from build123d import *

# Parameters (mm, degrees)
CUT_EXTRUDE1_DEPTH   = 5
CUT_EXTRUDE3_DEPTH   = 45
SKETCH8_R            = 40
CUT_EXTRUDE4_DEPTH   = 32
SKETCH9_R            = 32
SKETCH9_R_2          = 24.5
CUT_EXTRUDE5_DEPTH   = 14
SKETCH10_R           = 26
CUT_EXTRUDE6_DEPTH   = 14
FILLET1_R            = 7
FILLET2_R            = 7
CUT_REVOLVE1_START   = 22
CUT_REVOLVE1_DEPTH   = 30.5
CUT_EXTRUDE12_DEPTH  = 5
SKETCH18_W           = 13
SKETCH18_H           = 8
CUT_EXTRUDE13_DEPTH  = 5
INTERSECT1_OUTLINE_R = 42
INTERSECT1_DEPTH     = 55
SKETCH20_W           = 10
SKETCH20_H           = 5
BOSS_EXTRUDE1_DEPTH  = 13
BOSS_EXTRUDE3_DEPTH  = 7
SKETCH19_R           = 1.5
CUT_EXTRUDE14_DEPTH  = 20
SKETCH23_W           = 20
SKETCH23_H           = 7
CUT_EXTRUDE15_DEPTH  = 7
SKETCH24_W           = 44
SKETCH24_H           = 3.5
CUT_EXTRUDE16_DEPTH  = 5
SKETCH25_R           = 2.75
CUT_EXTRUDE17_DEPTH  = 5
FILLET4_R            = 3
FILLET6_R            = 4


with BuildPart() as part:
    # Sketch1 → Revolve1 (revolve)
    with BuildSketch(Plane.XY, mode=Mode.PRIVATE) as revolve1_sk:
        with BuildLine():
            Line((22.5, 0), (32, 0))
            ThreePointArc((32, 0), (33.414213562, 0.585786438), (34, 2))
            Line((34, 2), (34, 18))
            Line((34, 18), (40, 18))
            ThreePointArc((40, 18), (41.414213562, 18.585786438), (42, 20))
            Line((42, 20), (42, 55))
            ThreePointArc((42, 55), (40.535533906, 58.535533906), (37, 60))
            Line((37, 60), (0, 60))
            Line((0, 60), (0, 18))
            Line((0, 18), (22.5, 18))
            Line((22.5, 18), (22.5, 0))
        make_face()
    revolve(revolve1_sk.sketch.rotate(Axis((0, 2, 0), (0, 1, 0)), 90), axis=Axis((0, 2, 0), (0, 1, 0)))

    # Sketch5 → Cut-Extrude1 (cut)
    with BuildSketch(Plane(origin=(0, 60, 0), x_dir=(1, 0, 0), z_dir=(0, 1, 0))):
        with BuildLine():
            Line((-42, 0), (-40, 0))
            Line((-40, 0), (40, 0))
            Line((40, 0), (42, 0))
            ThreePointArc((42, 0), (0, 42), (-42, 0))
        make_face()
    extrude(amount=-CUT_EXTRUDE1_DEPTH, mode=Mode.SUBTRACT)

    # Sketch7 → Cut-Extrude3 (cut)
    with BuildSketch(Plane.XZ.offset(-18)):
        with BuildLine():
            Line((-21, 0), (21, 0))
            ThreePointArc((21, 0), (0, -21), (-21, 0))
        make_face()
    extrude(amount=-CUT_EXTRUDE3_DEPTH, mode=Mode.SUBTRACT)

    # Sketch8 → Cut-Extrude4 (cut)
    with BuildSketch(Plane(origin=(0, 52.5, 0), x_dir=(1, 0, 0), z_dir=(0, 1, 0))):
        with Locations(Location((0, 0, 0), (0, 0, 270))):
            Circle(SKETCH8_R)
        with BuildLine():
            Line((22.912878475, -2), (-22.912878475, -2))
            ThreePointArc((-22.912878475, -2), (0, 23), (22.912878475, -2))
        make_face(mode=Mode.SUBTRACT)
    extrude(amount=-CUT_EXTRUDE4_DEPTH, mode=Mode.SUBTRACT)

    # Sketch9 → Cut-Extrude5 (cut)
    with BuildSketch(Plane(origin=(0, 2, 0), x_dir=(-1, 0, 0), z_dir=(0, -1, 0))):
        with Locations(Location((0, 0, 0), (0, 0, 90))):
            Circle(SKETCH9_R)
        with Locations(Location((0, 0, 0), (0, 0, 90))):
            Circle(SKETCH9_R_2, mode=Mode.SUBTRACT)
    extrude(amount=-CUT_EXTRUDE5_DEPTH, mode=Mode.SUBTRACT)

    # Sketch10 → Cut-Extrude6 (cut)
    with BuildSketch(Plane(origin=(0, 2, 0), x_dir=(-1, 0, 0), z_dir=(0, -1, 0))):
        Circle(SKETCH10_R)
    extrude(amount=-CUT_EXTRUDE6_DEPTH, mode=Mode.SUBTRACT)

    # Fillet1
    fillet1_edges = [part.edges().sort_by_distance(p)[0] for p in [
        (21, 36.5, 0),
        (-21, 36.5, 0),
    ]]
    fillet(fillet1_edges, radius=FILLET1_R)

    # Fillet2
    fillet2_edges = [part.edges().sort_by_distance(p)[0] for p in [
        (-22.912878475, 36.5, 2),
        (22.912878475, 36.5, 2),
    ]]
    fillet(fillet2_edges, radius=FILLET2_R)

    # Cut-Revolve1: read off the stored shape, not the designer's step
    # Cut-Revolve1 outline → Cut-Revolve1 (cut)
    with BuildSketch(Plane(origin=(0, 0, 0), x_dir=(1, 0, 0), z_dir=(0, 1, 0)).offset(CUT_REVOLVE1_START)):
        with BuildLine():
            Line((-34.641016151, -20), (-36.373066959, -21))
            ThreePointArc((-36.373066959, -21), (0, -42), (36.373066959, -21))
            Line((36.373066959, -21), (34.641016151, -20))
            ThreePointArc((34.641016151, -20), (0, -40), (-34.641016151, -20))
        make_face()
    extrude(amount=CUT_REVOLVE1_DEPTH, mode=Mode.SUBTRACT)

    # Sketch15 → Cut-Extrude12 (cut)
    with BuildSketch(Plane(origin=(0, 20.5, 0), x_dir=(1, 0, 0), z_dir=(0, 1, 0))):
        with BuildLine():
            Line((-28.124355653, -3.514579578), (-26.124355653, -3.514579578))
            ThreePointArc((-26.124355653, -3.514579578), (-24.710142091, -2.928793141), (-24.124355653, -1.514579578))
            Line((-24.124355653, -1.514579578), (-24.124355653, 8.485420422))
            ThreePointArc((-24.124355653, 8.485420422), (-24.710142091, 9.899633984), (-26.124355653, 10.485420422))
            Line((-26.124355653, 10.485420422), (-28.124355653, 10.485420422))
            ThreePointArc((-28.124355653, 10.485420422), (-29.538569215, 9.899633984), (-30.124355653, 8.485420422))
            Line((-30.124355653, 8.485420422), (-30.124355653, -1.514579578))
            ThreePointArc((-30.124355653, -1.514579578), (-29.538569215, -2.928793141), (-28.124355653, -3.514579578))
        make_face()
    extrude(amount=-CUT_EXTRUDE12_DEPTH, mode=Mode.SUBTRACT)

    # Sketch18 → Cut-Extrude13 (cut)
    with BuildSketch(Plane(origin=(0, 55, 0), x_dir=(1, 0, 0), z_dir=(0, 1, 0))):
        with Locations((0.796512215, 32.951769165)):
            Rectangle(SKETCH18_W, SKETCH18_H)
    extrude(amount=-CUT_EXTRUDE13_DEPTH, mode=Mode.SUBTRACT)

    # Intersect1: read off the stored shape, not the designer's step
    # Intersect1 outline → Intersect1 (cut)
    with BuildSketch(Plane(origin=(0, 0, 0), x_dir=(1, 0, 0), z_dir=(0, 1, 0))):
        Circle(INTERSECT1_OUTLINE_R)
        with BuildLine():
            Line((12.124355653, 0), (-12.124355653, 0))
            ThreePointArc((-12.124355653, 0), (-18.186533479, 3.5), (-18.186533479, 10.5))
            ThreePointArc((-18.186533479, 10.5), (0, 21), (18.186533479, 10.5))
            ThreePointArc((18.186533479, 10.5), (18.186533479, 3.5), (12.124355653, 0))
        make_face(mode=Mode.SUBTRACT)
    extrude(amount=INTERSECT1_DEPTH, mode=Mode.SUBTRACT)

    # Sketch20 → Boss-Extrude1 (add)
    with BuildSketch(Plane.XZ.offset(-55)):
        with Locations((0, 30)):
            Rectangle(SKETCH20_W, SKETCH20_H)
    extrude(amount=BOSS_EXTRUDE1_DEPTH)

    # Sketch22 → Boss-Extrude3 (add)
    with BuildSketch(Plane(origin=(0, 0, 0), x_dir=(-1, 0, 0), z_dir=(0, 0, -1))):
        with BuildLine():
            Line((-42, 55), (42, 55))
            ThreePointArc((42, 55), (40.535533906, 58.535533906), (37, 60))
            Line((37, 60), (-37, 60))
            ThreePointArc((-37, 60), (-40.535533906, 58.535533906), (-42, 55))
        make_face()
    extrude(amount=BOSS_EXTRUDE3_DEPTH)

    # Sketch19 → Cut-Extrude14 (cut)
    with BuildSketch(Plane(origin=(0, 0, -7), x_dir=(-1, 0, 0), z_dir=(0, 0, -1))):
        with Locations((0, 57.5)):
            Circle(SKETCH19_R)
        with Locations((-29.45, 57.5)):
            Circle(SKETCH19_R)
        with Locations((29.45, 57.5)):
            Circle(SKETCH19_R)
    extrude(amount=-CUT_EXTRUDE14_DEPTH, mode=Mode.SUBTRACT)

    # Sketch23 → Cut-Extrude15 (cut)
    with BuildSketch(Plane(origin=(0, 60, 0), x_dir=(1, 0, 0), z_dir=(0, 1, 0))):
        with Locations((-32, 3.5)):
            Rectangle(SKETCH23_W, SKETCH23_H)
        with Locations((32, 3.5)):
            Rectangle(SKETCH23_W, SKETCH23_H)
    extrude(amount=-CUT_EXTRUDE15_DEPTH, mode=Mode.SUBTRACT)

    # Sketch24 → Cut-Extrude16 (cut)
    with BuildSketch(Plane(origin=(0, 60, 0), x_dir=(1, 0, 0), z_dir=(0, 1, 0))):
        with Locations((0, 5.25)):
            Rectangle(SKETCH24_W, SKETCH24_H)
    extrude(amount=-CUT_EXTRUDE16_DEPTH, mode=Mode.SUBTRACT)

    # Sketch25 → Cut-Extrude17 (cut)
    with BuildSketch(Plane(origin=(0, 0, 27.5), x_dir=(-1, 0, 0), z_dir=(0, 0, -1))):
        with Locations((0, 46.8)):
            Circle(SKETCH25_R)
    extrude(amount=-CUT_EXTRUDE17_DEPTH, mode=Mode.SUBTRACT)

    # Fillet4
    # the kernel refuses this fillet: 3 mm, written as the material it takes off along each edge
    with BuildSketch(Plane(origin=(12.5, 42, 27.5), x_dir=(0, 1, 0), z_dir=(-1, 0, 0))) as fillet4_piece_1:
        with BuildLine():
            CenterArc((FILLET4_R, -FILLET4_R), FILLET4_R, 90, 90)
            Line((0, -FILLET4_R), (0, 0))
            Line((0, 0), (FILLET4_R, 0))
        make_face()
    extrude(amount=25, mode=Mode.SUBTRACT)

    # Fillet6
    # the kernel refuses this fillet: 4 mm, written as the material it takes off along each edge
    with BuildSketch(Plane(origin=(-13.660254038, 42, 32.5), x_dir=(0, 1, 0), z_dir=(1, 0, 0))) as fillet6_piece_1:
        with BuildLine():
            CenterArc((3.464101615, -4), FILLET6_R, 90, 60)
            Line((0, -2), (0, 0))
            Line((0, 0), (3.464101615, 0))
        make_face()
    extrude(amount=27.320508076, mode=Mode.SUBTRACT)


solid = part.part
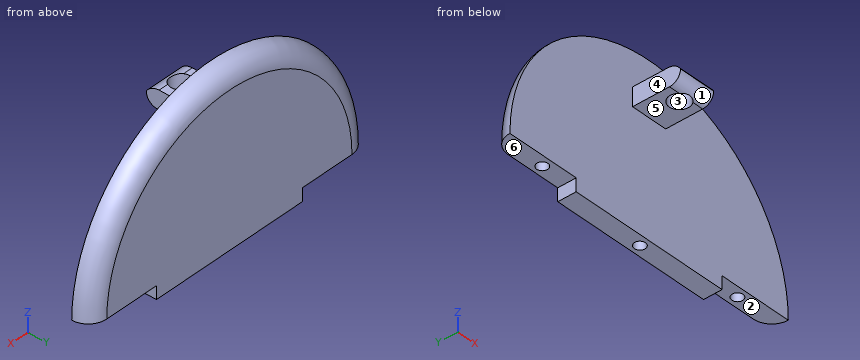
The model under review builds one solid part; all positions refer to its coordinate system, in mm. Face numbers are marked on the shaded views. A direction names the side the tool comes from. Round coordinates to 2 decimals unless told otherwise and drop trailing zeros. Loops run counter-clockwise (first coordinate to the right, second up) from the corner with the lowest first, then second, coordinate; pieces in that order, holes last. Notation, with made-up numbers: (83, -9.75) -> (133, -9.75) arc R16 cw to (133, -5.75) -> close; hole circle Ø5 at (-26.5, -9). An arc over 180 degrees is marked (long way). Answer as CSV lines item,"result".
1) Add section C-C on z = 9.5. State how many separate pieces and enclosed holes the cut face has, plus the area to 3 significant figures.
Geometry results:
separate pieces,"1"
enclosed holes,"3"
area,"377 mm²"
2) To check wall thickness, follow line 1 along Y through (x, z) = (0, 9); line 2 along Y through (x, z) = (-23, 12); line 3 along Y through (x, z) = (0, 29). State the ranges of each line that lie inside material, in increasing order. Write a range as from..to.
Geometry results:
line 1,"y = 55..56, 59..60"
line 2,"y = 55..60"
line 3,"y = 42.4..44.05, 49.55..60"
3) Add section A-A on y = 46.8. Write out the cut boundary in (x, z), plus the area to 3 significant figures.
Geometry results:
outline,"(-5, 27.5) -> (-2.75, 27.5) -> (-2.75, 32.5) -> (-5, 32.5) -> close; (2.75, 27.5) -> (5, 27.5) -> (5, 32.5) -> (2.75, 32.5) -> close"
area,"22.5 mm²"
4) Add section B-B on y = 52.75. Write out the cut boundary in (x, z), plus the area to 3 significant figures.
Geometry results:
outline,"(-5, 27.5) -> (5, 27.5) -> (5, 32.5) -> (-5, 32.5) -> close"
area,"50.0 mm²"
5) Tool access review of the marked faces 4, 5 and 6: name each direction out of +Z, -Z, +X, -X, +Y, -Y from which nothing blocks a thin tool from reaching the whole face with its end or side.
Geometry results:
face 4,"+Z, -Z, -X, -Y"
face 5,"-Z, +X, -X, -Y"
face 6,"-Z, -X, +Y, -Y"
6) For P1, Ø7, axis at x = 0, y = 46.8, coming from the +Z side; P2, Ø2.5, axis at y = 50, z = 30.5, coming from the -X side; P3, Ø2.5, axis at x = -30.5, y = 56.5, coming from the -Z side; P4, Ø5, axis at y = 50.5, z = 2.5, coming from the -X side, all flat-tipped, find the tip position at first contact; note any pin that passes through.
Geometry results:
P1,"stops at z = 32.5"
P2,"stops at x = -5"
P3,"stops at z = 0"
P4,"passes through"
7) Draft analysis for pull direction Y (two halves, no side actions). For the marked faces 1, 2 and 3, state which applies: pulls with the +Y half, pulls with the -Y half, needs draft (parallel to the pull), parting line crosses it, or undercut.
Geometry results:
face 1,"pulls with the -Y half"
face 2,"needs draft"
face 3,"undercut"
